```python
from build123d import *

# Parameters (mm, degrees)
SKETCH1_W           = 14.8
SKETCH1_H           = 68
BOSS_EXTRUDE1_DEPTH = 10
SKETCH2_W           = 8
SKETCH2_H           = 10
BOSS_EXTRUDE2_DEPTH = 40
FILLET2_R           = 3


with BuildPart() as part:
    # Sketch1 → Boss-Extrude1 (new body)
    with BuildSketch(Plane(origin=(0, 0, 0), x_dir=(1, 0, 0), z_dir=(0, 1, 0))):
        Rectangle(SKETCH1_W, SKETCH1_H)
    extrude(amount=BOSS_EXTRUDE1_DEPTH)

    # Sketch2 → Boss-Extrude2 (add)
    with BuildSketch(Plane.ZY.offset(7.4)):
        with Locations((-30, 5)):
            Rectangle(SKETCH2_W, SKETCH2_H)
    extrude(amount=BOSS_EXTRUDE2_DEPTH)

    # Fillet2
    fillet2_edges = [part.edges().sort_by_distance(p)[0] for p in [
        (-7.4, 5, -26),
        (-20, 10, -34),
        (-47.4, 5, -34),
        (-47.4, 5, -26),
        (-20, 0, -34),
        (7.4, 5, -34),
    ]]
    fillet(fillet2_edges, radius=FILLET2_R)


solid = part.part
```
CAD build for the part. Positions are in the model's coordinates, mm. A direction names the side the tool comes from. Coordinates: 2 decimals unless noted, no trailing zeros. Write each loop counter-clockwise with the first axis right and the second up, starting at its lowest first coordinate (ties: lowest second). Pieces come first, ordered by that corner, then holes.
(1) Cut at D-D, the plane x = -9.5. List the corners of the cut face in (y, z), and give its area (3 significant figures).
(2) 3-axis set-ups, long thin cutter, end or side, ignore diameter. For faces 1 (the face through (-46.838, 5.07, -32.748)), 2 (the face through (-27, 5, -26)): which of +Z, -Z, +X, -X, +Y, -Y reach the whole face in a straight line?
(3) Drill centre lines: probe 1 along X at (y, z) = (6, 25); probe 2 along Z at (x, y) = (4.5, 5.75); probe 3 along Z at (x, y) = (-31, 4.5). Where is each one in solid material? Low to high.
(4) Flat gauge pin, fed straight in: pin 1 (6 mm diameter, centred on y = 9, z = 23.5, fed in from -X). Where does the tip first touch, or does it go through?
(5) Cut at A-A, the plane y = 6. List the corners of the cut face in (x, z).
(6) Cut at B-B, the plane x = -42. List the corners of the cut face in (y, z).
(7) Cut at C-C, the plane z = 23. List the corners of the cut face in (x, y).
Geometry says:
1. outline: (0, -31) arc R3 ccw to (3, -34) - (7, -34) arc R3 ccw to (10, -31) - (10, -25.86) - (0, -25.86) - close
1. area: 77.5 mm2
2. face 1: -Z, -X, +Y, -Y
2. face 2: +Z, -X, +Y, -Y
3. probe 1: x = -7.4 to 7.4
3. probe 2: z = -34 to 34
3. probe 3: z = -34 to -26
4. pin 1: stops at x = -7.4
5. outline: (-47.4, -31) arc R3 ccw to (-44.4, -34) - (4.4, -34) arc R3 ccw to (7.4, -31) - (7.4, 34) - (-7.4, 34) - (-7.4, -23) arc R3 cw to (-10.4, -26) - (-44.4, -26) arc R3 ccw to (-47.4, -29) - close
6. outline: (0, -31) arc R3 ccw to (3, -34) - (7, -34) arc R3 ccw to (10, -31) - (10, -26) - (0, -26) - close
7. outline: (-7.4, 0) - (7.4, 0) - (7.4, 10) - (-7.4, 10) - close
